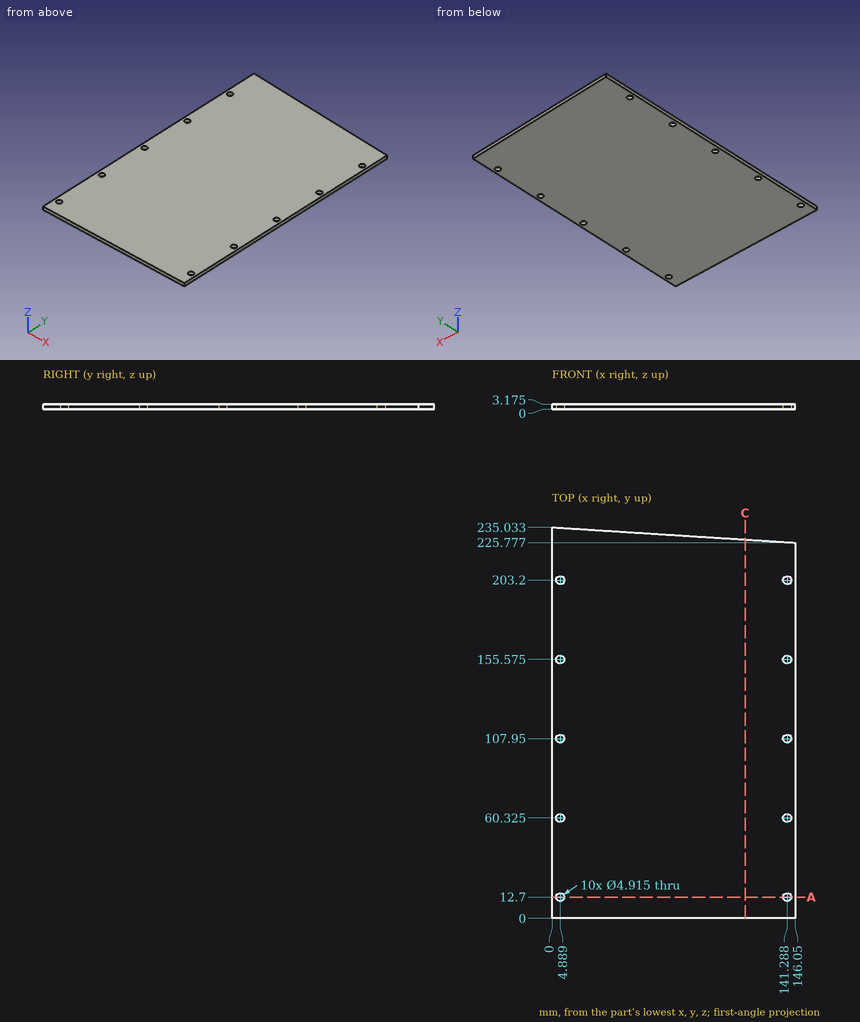
Answer from the drawing. Dimensions are ordinates in mm from the lowest x, y and z of the part. Give positions to 0.01 mm unless a question says otherwise; leave off trailing zeros. Write each loop counter-clockwise with the first axis right and the second up, starting at its lowest first coordinate (ties: lowest second). Pieces come first, ordered by that corner, then holes. Notation, with made-up numbers: (11, 35) -> (51, 35) arc R23 cw to (51, 68) -> close; hole circle Ø11 at (51, 21). An arc over 180 degrees is marked (long way). One line per question, with ' | ' between items. Start each with the question number.
1. Section C-C (x = 116) is taken. Determine the outline of the cut face in (y, z) (1 decimal).
2. Section A-A (y = 12.7) is taken. State how many separate pieces and enclosed holes the cut face has.
3. Find the intervals of material crossed by probe 1 along Y at (x, z) = (7, 1) (1 decimal); probe 2 along Y at (x, z) = (32, 1.5) (1 decimal); probe 3 along Y at (x, z) = (120.5, 2.9) (1 decimal), in increasing order.
Response values:
1) outline: (0, 0) -> (227.7, 0) -> (227.7, 3.2) -> (0, 3.2) -> close
2) separate pieces: 3 | enclosed holes: 0
3) probe 1: 0 to 11.4, 14 to 59.1, 61.6 to 106.7, 109.2 to 154.3, 156.8 to 201.9, 204.5 to 234.6 | probe 2: 0 to 233 | probe 3: 0 to 227.4
